from build123d import *

# Parameters (mm, degrees)
SKETCH1_R           = 44.45
BOSS_EXTRUDE1_DEPTH = 19.05
SKETCH2_W           = 8.414535341
SKETCH2_H           = 8.414535341
CUT_EXTRUDE1_DEPTH  = 29.972
CIRPATTERN1_COUNT   = 18
CUT_EXTRUDE2_DEPTH  = 6.35
FILLET3_R           = 3.81
CUT_EXTRUDE6_DEPTH  = 25.908


with BuildPart() as part:
    # Sketch1 → Boss-Extrude1 (new body)
    with BuildSketch(Plane(origin=(0, 0, 0), x_dir=(1, 0, 0), z_dir=(0, 1, 0))):
        with Locations(Location((0, 0, 0), (0, 0, 270))):
            Circle(SKETCH1_R)
    extrude(amount=BOSS_EXTRUDE1_DEPTH)

    # Sketch2 → Cut-Extrude1 (cut)
    with BuildSketch(Plane(origin=(0, 19.05, 0), x_dir=(1, 0, 0), z_dir=(0, 1, 0))):
        with Locations((-31.148036033, 31.148036033)):
            Rectangle(SKETCH2_W, SKETCH2_H)
    cut_extrude1 = extrude(amount=-CUT_EXTRUDE1_DEPTH, mode=Mode.SUBTRACT)

    # CirPattern1: Cut-Extrude1 ×18 about axis
    cirpattern1_axis = Axis((0, 0, 0), (0, 1, 0))
    for i in range(1, CIRPATTERN1_COUNT):
        add(cut_extrude1.rotate(cirpattern1_axis, i * 360 / CIRPATTERN1_COUNT), mode=Mode.SUBTRACT)

    # Sketch4 → Cut-Extrude2 (cut)
    with BuildSketch(Plane.XZ):
        Polygon((4.671980957, -17.436070304), (14.786635004, -10.353713294), (17.982458197, 1.573261235), (12.764089347, 12.764089347), (1.573261235, 17.982458197), (-10.353713294, 14.786635004), (-17.436070304, 4.671980957), (-16.359896238, -7.628744902), (-7.628744902, -16.359896238), align=None)
    extrude(amount=-CUT_EXTRUDE2_DEPTH, mode=Mode.SUBTRACT)

    # Fillet3
    # the kernel refuses this fillet: 3.81 mm, written as the material it takes off along each edge
    with BuildSketch(Plane(origin=(-9.766541838, 24.122461368, -43.363777056), x_dir=(-0.9702942077465824, 0, 0.24192798600705953), z_dir=(0, -1, 0)), Plane(origin=(-24.008832539, 24.122461368, -37.408267269), x_dir=(-0.8290340625621466, 0, 0.5591981072139847), z_dir=(0, -1, 0)), Plane(origin=(-35.355303704, 24.122461368, -26.940768363), x_dir=(-0.5877801741930432, 0, 0.8090206838057948), z_dir=(0, -1, 0)), Plane(origin=(35.355303704, 24.122461368, 26.940768363), x_dir=(0.5877801741930427, 0, -0.8090206838057951), z_dir=(0, -1, 0)), Plane(origin=(42.437403453, 24.122461368, 13.223815189), x_dir=(0.2756313221047677, 0, -0.9612634260569668), z_dir=(0, -1, 0)), Plane(origin=(44.400926037, 24.122461368, -2.08812526), x_dir=(-0.06976273531441618, 0, -0.9975636123884285), z_dir=(0, -1, 0)), Plane(origin=(41.009041652, 24.122461368, -17.148206985), x_dir=(-0.40674237726635254, 0, -0.913542904594916), z_dir=(0, -1, 0)), Plane(origin=(32.670861615, 24.122461368, -30.139961867), x_dir=(-0.6946628856418128, 0, -0.7193354400499046), z_dir=(0, -1, 0)), Plane(origin=(20.392093497, 24.122461368, -39.496392529), x_dir=(-0.8987967978765562, 0, -0.43836550517444806), z_dir=(0, -1, 0)), Plane(origin=(5.653737948, 24.122461368, -44.088975348), x_dir=(-0.9945225514593977, 0, -0.10452222078911967), z_dir=(0, -1, 0))) as fillet3_piece_1:
        with BuildLine():
            CenterArc((1.942028067, -3.809007557), FILLET3_R, 88.692212078, 55.30814756)
            Line((-1.140340739, -1.569565093), (0, 0))
            ThreePointArc((0, 0), (1.014492274, 0.0115785), (2.028984547, 0))
        make_face()
    extrude(amount=29.194922737, mode=Mode.SUBTRACT)
    with BuildSketch(Plane(origin=(-13.223815189, 24.122461368, -42.437403453), x_dir=(-0.34202014332566844, 0, 0.9396926207859085), z_dir=(0, -1, 0)), Plane(origin=(-26.940768363, 24.122461368, -35.355303704), x_dir=(0, 0, 1), z_dir=(0, -1, 0)), Plane(origin=(37.408267269, 24.122461368, 24.008832539), x_dir=(-0.3420201433256682, 0, -0.9396926207859086), z_dir=(0, -1, 0)), Plane(origin=(43.363777056, 24.122461368, 9.766541838), x_dir=(-0.6427876096865393, 0, -0.7660444431189782), z_dir=(0, -1, 0)), Plane(origin=(44.088975348, 24.122461368, -5.653737948), x_dir=(-0.8660254037844388, 0, -0.4999999999999997), z_dir=(0, -1, 0)), Plane(origin=(39.496392529, 24.122461368, -20.392093497), x_dir=(-0.984807753012208, 0, -0.1736481776669302), z_dir=(0, -1, 0)), Plane(origin=(30.139961867, 24.122461368, -32.670861615), x_dir=(-0.9848077530122079, 0, 0.17364817766693105), z_dir=(0, -1, 0)), Plane(origin=(17.148206985, 24.122461368, -41.009041652), x_dir=(-0.8660254037844395, 0, 0.49999999999999856), z_dir=(0, -1, 0)), Plane(origin=(2.08812526, 24.122461368, -44.400926037), x_dir=(-0.6427876096865408, 0, 0.7660444431189768), z_dir=(0, -1, 0))) as fillet3_piece_2:
        with BuildLine():
            CenterArc((1.940080303, -3.81), FILLET3_R, 90, 55.30814756)
            ThreePointArc((-1.192596891, -1.641490466), (-0.605665691, -0.81393962), (0, 0))
            Line((0, 0), (1.940080303, 0))
        make_face()
    extrude(amount=29.194922737, mode=Mode.SUBTRACT)
    with BuildSketch(Plane(origin=(-37.408267269, 24.122461368, -24.008832539), x_dir=(0.559198107213983, 0, -0.8290340625621475), z_dir=(0, -1, 0)), Plane(origin=(-43.363777056, 24.122461368, -9.766541838), x_dir=(0.24192798600706303, 0, -0.9702942077465815), z_dir=(0, -1, 0)), Plane(origin=(-44.088975348, 24.122461368, 5.653737948), x_dir=(-0.1045222207891241, 0, -0.9945225514593973), z_dir=(0, -1, 0)), Plane(origin=(-39.496392529, 24.122461368, 20.392093497), x_dir=(-0.43836550517444245, 0, -0.8987967978765589), z_dir=(0, -1, 0)), Plane(origin=(-30.139961867, 24.122461368, 32.670861615), x_dir=(-0.7193354400499047, 0, -0.6946628856418126), z_dir=(0, -1, 0)), Plane(origin=(-17.148206985, 24.122461368, 41.009041652), x_dir=(-0.9135429045949142, 0, -0.4067423772663572), z_dir=(0, -1, 0)), Plane(origin=(-2.08812526, 24.122461368, 44.400926037), x_dir=(-0.9975636123884287, 0, -0.06976273531441333), z_dir=(0, -1, 0)), Plane(origin=(13.223815189, 24.122461368, 42.437403453), x_dir=(-0.9612634260569665, 0, 0.2756313221047693), z_dir=(0, -1, 0)), Plane(origin=(26.940768363, 24.122461368, 35.355303704), x_dir=(-0.809020683805795, 0, 0.587780174193043), z_dir=(0, -1, 0))) as fillet3_piece_3:
        with BuildLine():
            CenterArc((1.942028067, 3.809007557), FILLET3_R, 215.999640362, 55.30814756)
            Line((-1.140340739, 1.569565093), (0, 0))
            ThreePointArc((0, 0), (1.014492274, -0.0115785), (2.028984547, 0))
        make_face()
    extrude(amount=29.194922737, mode=Mode.SUBTRACT)
    with BuildSketch(Plane(origin=(-42.437403453, 24.122461368, -13.223815189), x_dir=(0.9396926207859084, 0, -0.3420201433256688), z_dir=(0, -1, 0)), Plane(origin=(-44.400926037, 24.122461368, 2.08812526), x_dir=(0.7660444431189783, 0, -0.6427876096865389), z_dir=(0, -1, 0)), Plane(origin=(-41.009041652, 24.122461368, 17.148206985), x_dir=(0.4999999999999989, 0, -0.8660254037844393), z_dir=(0, -1, 0)), Plane(origin=(-32.670861615, 24.122461368, 30.139961867), x_dir=(0.173648177666932, 0, -0.9848077530122078), z_dir=(0, -1, 0)), Plane(origin=(-20.392093497, 24.122461368, 39.496392529), x_dir=(-0.17364817766693083, 0, -0.9848077530122079), z_dir=(0, -1, 0)), Plane(origin=(-5.653737948, 24.122461368, 44.088975348), x_dir=(-0.49999999999999867, 0, -0.8660254037844395), z_dir=(0, -1, 0)), Plane(origin=(9.766541838, 24.122461368, 43.363777056), x_dir=(-0.7660444431189792, 0, -0.6427876096865378), z_dir=(0, -1, 0)), Plane(origin=(24.008832539, 24.122461368, 37.408267269), x_dir=(-0.9396926207859089, 0, -0.34202014332566766), z_dir=(0, -1, 0))) as fillet3_piece_4:
        with BuildLine():
            CenterArc((1.940080303, 3.81), FILLET3_R, 214.69185244, 55.30814756)
            ThreePointArc((-1.192596891, 1.641490466), (-0.605665691, 0.81393962), (0, 0))
            Line((0, 0), (1.940080303, 0))
        make_face()
    extrude(amount=29.194922737, mode=Mode.SUBTRACT)

    # Sketch6 → Cut-Extrude6 (cut)
    with BuildSketch(Plane(origin=(0, 19.05, 0), x_dir=(1, 0, 0), z_dir=(0, 1, 0))):
        Polygon((3.666174209, 0), (1.833087105, 3.175), (-1.833087105, 3.175), (-3.666174209, 0), (-1.833087105, -3.175), (1.833087105, -3.175), align=None)
    extrude(amount=-CUT_EXTRUDE6_DEPTH, mode=Mode.SUBTRACT)


solid = part.part
Part model, mm, in its own coordinate system. A direction names the side the tool comes from. Coordinates: 2 decimals unless noted, no trailing zeros. Put each result on its own line as item: value.
1. Two-plate mould, pull along Z, no slides. Class faces 1 (the flat face through (0, 6.35, -3.4)), 2 (the flat face through (2.76, 12.79, -1.57)), 3 (the cylindrical face through (-20.051, 9.658, 39.175)), 4 (the cylindrical face through (20.051, 9.658, -39.175)): +Z half, -Z half, draft (parallel to the pull), parting line (faces both ways), or undercut.
Final values:
face 1: undercut
face 2: undercut
face 3: +Z half
face 4: -Z half
2. 3-axis set-ups, long thin cutter, end or side, ignore diameter. For faces 5 (the flat face through (19.186, 9.658, 35.653)), 6 (the flat face through (-34.35, 9.66, 21.3)), 7 (the flat face through (40.01, 9.66, 5.77)): which of +Z, -Z, +X, -X, +Y, -Y reach the whole face in a straight line?
Final values:
face 5: +Z, +Y, -Y
face 6: -X, +Y, -Y
face 7: +X, +Y, -Y
3. Flat gauge pins, fed straight in: pin 1 Ø3 at (x, y) = (-0.5, 14) entering from -Z; pin 2 Ø1.5 at (x, y) = (-1.5, 10.5) entering from +Z; pin 3 Ø4 at (x, y) = (-20, 13.5) entering from -Z; pin 4 Ø5 at (x, z) = (-22.5, -1) entering from -Y. Where does each tip first touch, or does it go through?
Final values:
pin 1: stops at z = -43.09
pin 2: stops at z = 43.96
pin 3: stops at z = -36.68
pin 4: stops at y = 0
4. Probe line 1 along Z through (x, y) = (-40, 18.25); line 2 along X through (y, z) = (13.5, -29); line 3 along Z through (x, y) = (-6.5, 4). List the from-to ranges inside material, lowest first. Write a range as [from, to].
Final values:
line 1: z = [-14.11, -5.76], [-1.6, 8.01], [15.4, 19.23]
line 2: x = [-26.94, 32.39]
line 3: z = [-40.62, -16.46], [15.82, 42.61]
